Model file for the job. Use its own axes, mm. A direction names the side the tool comes from. Round coordinates to 2 decimals unless told otherwise and drop trailing zeros. Order: outer loops, then holes, each group sorted by start corner. A loop starts at its lowest first (then second) coordinate and runs counter-clockwise, first axis right, second up. Notation, with made-up numbers: (89.25, 87) - (142.25, 87) arc R21 cw to (142.25, 108) - close; hole circle Ø11 at (18.5, 12). An arc over 180 degrees is marked (long way). Use one line per item in the form item = value.
from build123d import *

# Parameters (mm, degrees)
SKETCH_1_W      = 30
SKETCH_1_H      = 5
EXTRUDE_1_DEPTH = 5


with BuildPart() as part:
    # 草图1 → 凸台-拉伸1 (new body)
    with BuildSketch(Plane.XY):
        Polygon((0, 75), (0, 83), (30, 83), (30, 88), (70, 88), (70, 83), (100, 83), (100, 75), (105, 75), (105, 55), (100, 55), (100, 30), (105, 30), (105, 10), (100, 10), (100, 0), (0, 0), (0, 10), (-5, 10), (-5, 30), (0, 30), (0, 55), (-5, 55), (-5, 75), align=None)
        with Locations((30, 43)):
            Rectangle(SKETCH_1_W, SKETCH_1_H, mode=Mode.SUBTRACT)
    extrude(amount=EXTRUDE_1_DEPTH)


solid = part.part
(1) Slice it at D-D on y = 31.5. Give the cut face in (x, z).
Report:
outline = (0, 0) - (100, 0) - (100, 5) - (0, 5) - close
(2) Slice it at B-B on y = 43. Give the cut face in (x, z), then the cut area to 3 significant figures.
Report:
outline = (0, 0) - (15, 0) - (15, 5) - (0, 5) - close; (45, 0) - (100, 0) - (100, 5) - (45, 5) - close
area = 350 mm2
(3) Pin check, flat tips, straight feed: pin 1 (2.5 mm diameter, centred on y = 42, z = 3, fed in from +X); pin 2 (2.5 mm diameter, centred on y = 6, z = 1.5, fed in from -X); pin 3 (1.5 mm diameter, centred on x = 103, z = 2, fed in from +Y). Stop position of each tip, or through.
Report:
pin_1 = 100
pin_2 = 0
pin_3 = 75
(4) Slice it at A-A on x = 28.5. Give the cut face in (y, z), then the cut area to 3 significant figures.
Report:
outline = (0, 0) - (40.5, 0) - (40.5, 5) - (0, 5) - close; (45.5, 0) - (83, 0) - (83, 5) - (45.5, 5) - close
area = 390 mm2
(5) Slice it at C-C on z = 3.7. Give the cut face in (x, y), then the cut area to 3 significant figures.
Report:
outline = (-5, 10) - (0, 10) - (0, 0) - (100, 0) - (100, 10) - (105, 10) - (105, 30) - (100, 30) - (100, 55) - (105, 55) - (105, 75) - (100, 75) - (100, 83) - (70, 83) - (70, 88) - (30, 88) - (30, 83) - (0, 83) - (0, 75) - (-5, 75) - (-5, 55) - (0, 55) - (0, 30) - (-5, 30) - close; hole (15, 40.5) - (45, 40.5) - (45, 45.5) - (15, 45.5) - close
area = 8,750 mm2
(6) Tool access for faces 1 (the face through (103, 10, 2)), 2 (the face through (-3, 30, 2)), 3 (the face through (0, 79, 2)), 4 (the face through (100, 79, 2)): list every direction of +Z, -Z, +X, -X, +Y, -Y with a clear straight run to the whole face (end or side of a thin tool).
Report:
face_1 = +Z, -Z, +X, -Y
face_2 = +Z, -Z, -X
face_3 = +Z, -Z, -X, +Y
face_4 = +Z, -Z, +X, +Y
(7) Probe probe 1 along X at (y, z) = (41, 0.8); probe 2 along Y at (x, z) = (29, 4.05); probe 3 along Y at (x, z) = (33, 3.65). List the from-to ranges inside material, lowest first. Write a range as [from, to].
Report:
probe_1 = [0, 15], [45, 100]
probe_2 = [0, 40.5], [45.5, 83]
probe_3 = [0, 40.5], [45.5, 88]
(8) Pull direction Y, two halves, no side cores. Call faces 5 (the face through (51, 0, 2)), 6 (the face through (30, 40.5, 2)), 7 (the face through (105, 65, 2)): released by +Y, released by -Y, zero draft, split by the parting line, or undercut.
Report:
face_5 = released by -Y
face_6 = undercut
face_7 = zero draft
